Can you work these out from the model? Positions are in its coordinate system, mm. Give positions to 0.01 mm unless a question says otherwise; leave off trailing zeros.
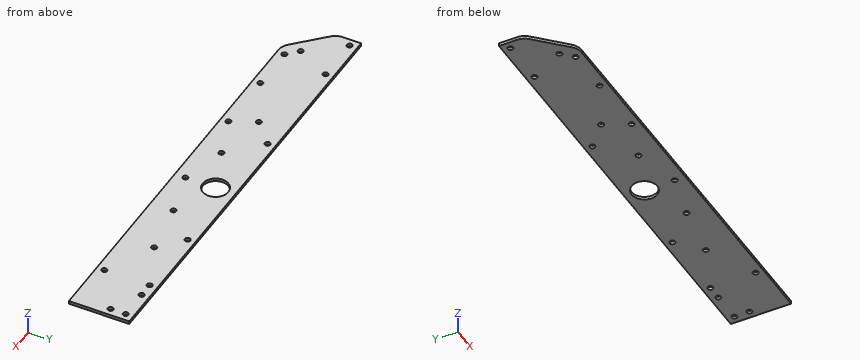
from build123d import *

# Parameters (mm, degrees)
SKETCH1_W           = 368.3
SKETCH1_H           = 50.8
SKETCH1_R           = 2.286
SKETCH1_R_2         = 10.795
BOSS_EXTRUDE1_DEPTH = 2.54
CUT_EXTRUDE1_DEPTH  = 2.54
FILLET1_R           = 12.7
SKETCH4_R           = 2.286
CUT_EXTRUDE3_DEPTH  = 372.795618048
SKETCH5_R           = 2.286
CUT_EXTRUDE4_DEPTH  = 372.795618048


with BuildPart() as part:
    # Sketch1 → Boss-Extrude1 (new body)
    with BuildSketch(Plane.XY):
        with Locations((-184.15, 25.4)):
            Rectangle(SKETCH1_W, SKETCH1_H)
        with Locations((-44.45, 6.35)):
            Circle(SKETCH1_R, mode=Mode.SUBTRACT)
        with Locations((-292.1, 6.35)):
            Circle(SKETCH1_R, mode=Mode.SUBTRACT)
        with Locations((-130.175, 19.05)):
            Circle(SKETCH1_R, mode=Mode.SUBTRACT)
        with Locations((-206.375, 19.05)):
            Circle(SKETCH1_R, mode=Mode.SUBTRACT)
        with Locations((-168.275, 34.29)):
            Circle(SKETCH1_R_2, mode=Mode.SUBTRACT)
        with Locations((-251.333, 26.67)):
            Circle(SKETCH1_R, mode=Mode.SUBTRACT)
        with Locations(Location((-85.217, 26.67, 0), (0, 0, 180))):
            Circle(SKETCH1_R, mode=Mode.SUBTRACT)
        with Locations((-330.2, 6.35)):
            Circle(SKETCH1_R, mode=Mode.SUBTRACT)
        with Locations((-241.3, 6.35)):
            Circle(SKETCH1_R, mode=Mode.SUBTRACT)
        with Locations((-361.95, 44.45)):
            Circle(SKETCH1_R, mode=Mode.SUBTRACT)
        with Locations((-323.85, 44.45)):
            Circle(SKETCH1_R, mode=Mode.SUBTRACT)
        with Locations((-339.180256121, 15.330256121)):
            Circle(SKETCH1_R, mode=Mode.SUBTRACT)
    extrude(amount=BOSS_EXTRUDE1_DEPTH)

    # Sketch2 → Cut-Extrude1 (cut)
    with BuildSketch(Plane.XY.offset(2.54)):
        Polygon((-388.62, 50.8), (-337.82, 0), (-388.62, 0), align=None)
    extrude(amount=-CUT_EXTRUDE1_DEPTH, mode=Mode.SUBTRACT)

    # Fillet1
    fillet1_edges = [part.edges().sort_by_distance(p)[0] for p in [
        (-337.82, 0, 1.27),
        (-368.3, 30.48, 1.27),
    ]]
    fillet(fillet1_edges, radius=FILLET1_R)

    # Sketch4 → Cut-Extrude3 (cut, through all)
    with BuildSketch(Plane.XY.offset(2.54)):
        with Locations((-231.775, 44.45)):
            Circle(SKETCH4_R)
        with Locations((-104.775, 44.45)):
            Circle(SKETCH4_R)
        with Locations((-168.275, 8.89)):
            Circle(SKETCH4_R)
    extrude(amount=-CUT_EXTRUDE3_DEPTH, mode=Mode.SUBTRACT)

    # Sketch5 → Cut-Extrude4 (cut, through all)
    with BuildSketch(Plane.XY.offset(2.54)):
        with Locations((-44.45, 44.45)):
            Circle(SKETCH5_R)
        with Locations((-31.75, 44.45)):
            Circle(SKETCH5_R)
        with Locations((-6.35, 44.45)):
            Circle(SKETCH5_R)
        with Locations((-6.35, 31.75)):
            Circle(SKETCH5_R)
    extrude(amount=-CUT_EXTRUDE4_DEPTH, mode=Mode.SUBTRACT)


solid = part.part
(1) Suppose I cut it at A-A on z = 2.05. Give the number of separate pieces and of enclosed holes in the cut face, plus the area to 3 significant figures.
Returned:
separate pieces: 1
enclosed holes: 19
area: 17,600 mm2
(2) Will this pin go through, and if not, where does the flat tip stop? P1, Ø3.5, axis at x = -231.775, y = 44.45, coming from the -Z side.
Returned:
P1: passes through
(3) Please list where these lines run through material, in increasing order: probe 1 along Y at (x, z) = (-241.3, 0.9); probe 2 along X at (y, z) = (8, 0.6); probe 3 along X at (y, z) = (18.5, 2.35).
Returned:
probe 1: y = 0 to 4.06, 8.64 to 50.8
probe 2: x = -345.82 to -331.78, -328.62 to -293.68, -290.52 to -242.88, -239.72 to -170.38, -166.17 to -46.03, -42.87 to 0
probe 3: x = -356.32 to -208.59, -204.16 to -132.39, -127.96 to 0
